Design review of the part built by this model. Coordinates are the model's own, in mm. Face numbers are marked on the shaded views. Give positions to 0.01 mm unless a question says otherwise; leave off trailing zeros. Loops run counter-clockwise (first coordinate to the right, second up) from the corner with the lowest first, then second, coordinate; pieces in that order, holes last. Notation, with made-up numbers: (29, 46.5) - (63, 46.5) arc R38 cw to (63, 85.5) - close; hole circle Ø8 at (-3.5, -2). An arc over 180 degrees is marked (long way). Write each question's results on one line, items separated by ' | '.
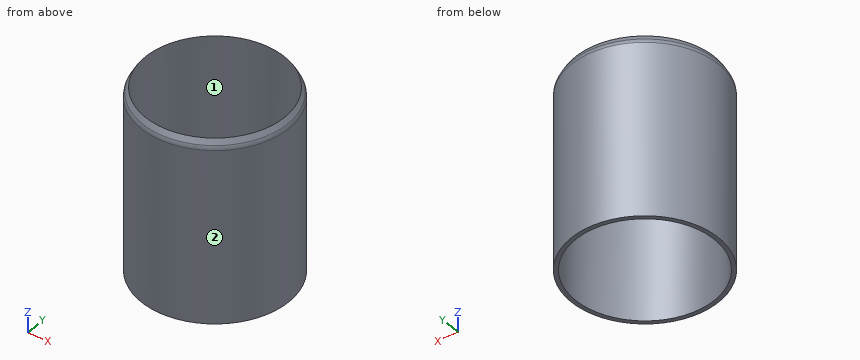
from build123d import *

# Parameters (mm, degrees)
F0_R     = 22.25
F0_R_2   = 21
F1_DEPTH = 55
F2_SIZE2 = 2.165054
F2_SIZE  = 1.24999
F3_R     = 2.5


# Not quite as in the source:
# - a fillet or chamfer is up to 0.001 mm smaller than in the source, because OpenCascade refuses the exact size


with BuildPart() as f1:
    # F0 (on Top) → F1 (new body)
    with BuildSketch(Plane.XY):
        Circle(F0_R)
        Circle(F0_R_2, mode=Mode.SUBTRACT)
    extrude(amount=F1_DEPTH)

    # F2 (size 1.25 and 2.1650635095 in the source; OpenCascade refuses exactly that, so slightly less here)
    f2_edges = [f1.edges().sort_by_distance(p)[0] for p in [
        (-22.25, 0, 55),
    ]]
    f2_side = f1.faces().sort_by_distance((-21.620675, 0, 55))[0]
    chamfer(f2_edges, length=F2_SIZE, length2=F2_SIZE2, reference=f2_side)

    # F3
    f3_edges = [f1.edges().sort_by_distance(p)[0] for p in [
        (-22.25, 0, 52.834946),
    ]]
    fillet(f3_edges, radius=F3_R)


solid = f1.part
(1) Take a section at A-A on z = 10.5. Give the boundary of the cut face in (x, y).
Answers below:
outline: circle Ø44.5 at (0, 0); hole circle Ø42 at (0, 0)
(2) Insertion check: P1, Ø10, axis at x = 4, y = -12, coming from the -Z side; P2, Ø2, axis at x = -17, z = 49.5, coming from the -Y side; P3, Ø1, axis at y = 17, z = 24.5, coming from the -X side; P4, Ø3, axis at x = -11, z = 8.5, coming from the +Y side. Each pin has a flat end and moves straight along its axis. Give the tip position at first contact, or say it passes through.
Answers below:
P1: through | P2: y = -15.46 | P3: x = -14.93 | P4: y = 20.12
(3) Wall thickness on line 1 along Y through (x, z) = (0, 27); line 2 along X through (y, z) = (16, 9.5); line 3 along Y through (x, z) = (-10, 47.5): over which ranges is each line inside the solid? List them lowest first. Write a range as from..to.
Answers below:
line 1: -22.25..-21, 21..22.25 | line 2: -15.46..-13.6, 13.6..15.46 | line 3: -19.88..-18.47, 18.47..19.88
(4) Draft analysis for pull direction X (two halves, no side actions). For the marked faces 1 and 2, state which applies: pulls with the +X half, pulls with the -X half, needs draft (parallel to the pull), parting line crosses it, or undercut.
Answers below:
face 1: undercut | face 2: parting line crosses it
